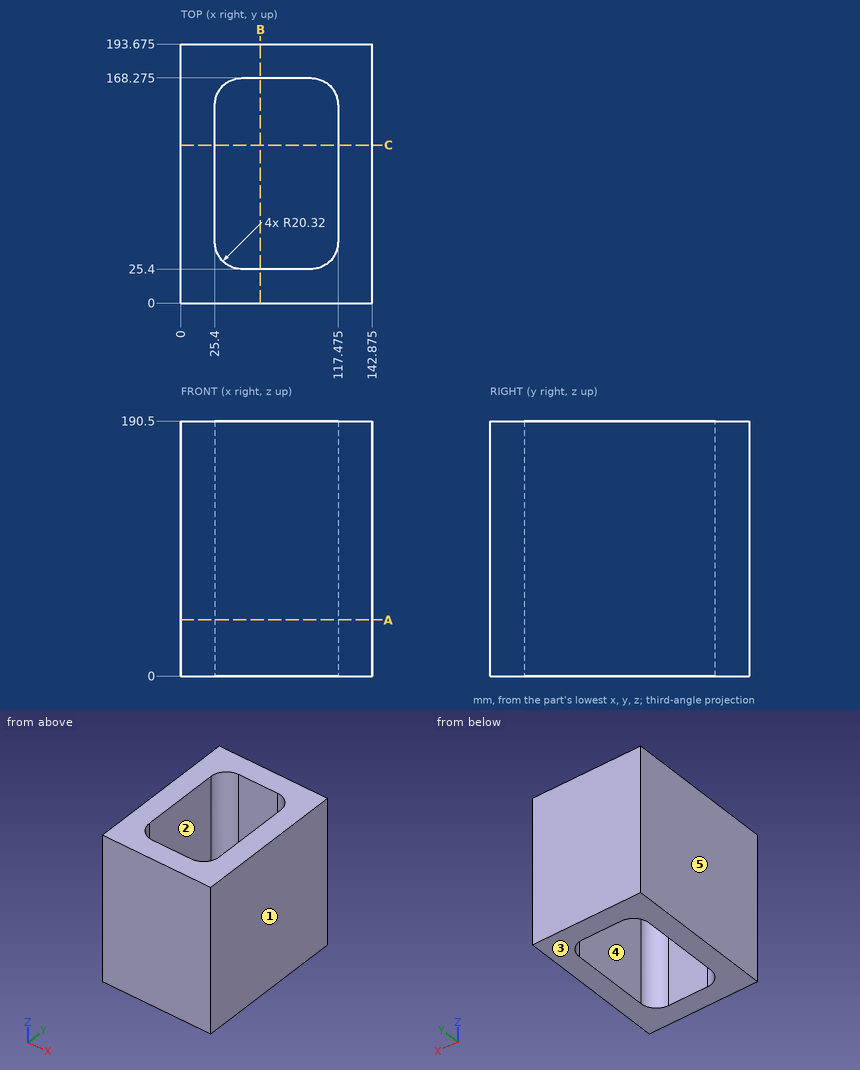
Verification items for this drawing (mm, ordinates from the low corner). A direction names the side the tool comes from. Coordinates: 2 decimals unless noted, no trailing zeros. Loops run counter-clockwise (first coordinate to the right, second up) from the corner with the lowest first, then second, coordinate; pieces in that order, holes last. Notation, with made-up numbers: (-2.75, 89) - (33.25, 89) arc R35 ccw to (33.25, 125) - close; hole circle Ø3 at (33, -28). An arc over 180 degrees is marked (long way). One line per item, written item: value. Start each with the question number.
(1) Material ranges on line 1 (Y direction, x = 59.5, z = 150) (3 decimals); line 2 (X direction, y = 139, z = 136.5) (3 decimals); line 3 (Y direction, x = 44.5, z = 163) (3 decimals), recorded low to high. Write a range as [from, to].
(2) Cross-section at A-A on z = 42. Enter the section's corners in (x, y) (3 decimals), plus the area to 3 significant figures.
(3) Tool access check on the marked faces 4 and 5. Record the directions out of +Z, -Z, +X, -X, +Y, -Y that give a thin tool (end or side, any length) a straight path to the whole face; none if there is none.
(4) Cross-section at B-B on x = 59.5. Enter the section's corners in (y, z) (3 decimals), plus the area to 3 significant figures.
(5) Cross-section at C-C on y = 118. Enter the section's corners in (x, z) (3 decimals).
(6) Mould release check, pull along X, two halves, no side actions. Record for the marked faces 1, 2 and 3: released by +X, released by -X, zero draft, split by the parting line, or undercut.
Results below:
1. line 1: y = [0, 25.4], [168.275, 193.675]
1. line 2: x = [0, 25.4], [117.475, 142.875]
1. line 3: y = [0, 25.437], [168.238, 193.675]
2. outline: (0, 0) - (142.875, 0) - (142.875, 193.675) - (0, 193.675) - close; hole (25.4, 45.72) arc R20.32 ccw to (45.72, 25.4) - (97.155, 25.4) arc R20.32 ccw to (117.475, 45.72) - (117.475, 147.955) arc R20.32 ccw to (97.155, 168.275) - (45.72, 168.275) arc R20.32 ccw to (25.4, 147.955) - close
2. area: 14,900 mm2
3. face 4: +Z, -Z
3. face 5: +Z, -Z, -X, +Y, -Y
4. outline: (0, 0) - (25.4, 0) - (25.4, 190.5) - (0, 190.5) - close; (168.275, 0) - (193.675, 0) - (193.675, 190.5) - (168.275, 190.5) - close
4. area: 9,680 mm2
5. outline: (0, 0) - (25.4, 0) - (25.4, 190.5) - (0, 190.5) - close; (117.475, 0) - (142.875, 0) - (142.875, 190.5) - (117.475, 190.5) - close
6. face 1: released by +X
6. face 2: undercut
6. face 3: zero draft
